Here's how the part is built. I have some questions about the finished solid (model axes, mm). A direction names the side the tool comes from. Coordinates: 2 decimals unless noted, no trailing zeros. Order: outer loops, then holes, each group sorted by start corner. A loop starts at its lowest first (then second) coordinate and runs counter-clockwise, first axis right, second up. Notation, with made-up numbers: (-1, 43.5) - (55, 43.5) arc R17 cw to (55, 52.5) - close; hole circle Ø3 at (84, 29.25). An arc over 180 degrees is marked (long way). Answer in a Markdown table with one row per item. Add a question column.
Item 1: Thinking about a two-plate mould opening in X: for faces 4 (the flat face through (42, 1, -32.5)), 5 (the flat face through (19, 1, -30)), 6 (the cylindrical face through (47.657, 1.47, -40.52)), which applies, +X half, -X half, draft (parallel to the pull), parting line (faces both ways), or undercut?
Item 2: I want a section at B-B (x = -24). Please give me the cut outline in (y, z), plus the area to 3 significant figures.
Item 3: Will these pins go through, and if not, where does the flat tip stop? pin 1 Ø7.5 at (x, z) = (50, -40) entering from +Y; pin 2 Ø0.9 at (x, y) = (35, 1) entering from +Z; pin 3 Ø0.9 at (y, z) = (1, -34) entering from +X; pin 4 Ø1.5 at (x, y) = (20, 2) entering from -Z.
Item 4: I want a section at C-C (y = 1.15). Please give me the cut outline in (x, z).
Item 5: If I drill on line 1 along X through (y, z) = (2.45, -46.5); line 2 along X through (y, z) = (1.15, -53); line 3 along X through (y, z) = (2.7, -38), over which ranges is the centre line in solid material (lowest first)? Write a range as from..to.
Item 6: On a 3-axis mill with a long thin cutter (end or side, diameter ignored), from which of +Z, -Z, +X, -X, +Y, -Y can I reach the whole of each face in a straight line? I mean faces 1 (the flat face through (0, 1, -45.2)), 2 (the cylindrical face through (1.13, 1.43, -72.99)), 3 (the flat face through (-43, 1, -32.5)). Say none if no direction works.
Item 7: I want a section at D-D (z = -40.5). Please give me the cut outline in (x, y), plus the area to 3 significant figures.
Item 8: I want a section at A-A (z = -48). Please give me the cut outline in (x, y).
```python
from build123d import *

# Parameters (mm, degrees)
BOSS_EXTRUDE1_DEPTH  = 2.9
SOLENOID_PLACEMENT_W = 38
SOLENOID_PLACEMENT_H = 64
CUT_EXTRUDE1_DEPTH   = 104.278313309
CUT_EXTRUDE4_DEPTH   = 104.278313309
SKETCH5_R            = 12
CUT_EXTRUDE5_DEPTH   = 104.278313309
SKETCH6_R            = 2.4
CUT_EXTRUDE6_DEPTH   = 104.278313309
CUT_EXTRUDE3_DEPTH   = 104.278313309


with BuildPart() as part:
    # Sketch1 → Boss-Extrude1 (new body)
    with BuildSketch(Plane(origin=(0, 0, 0), x_dir=(1, 0, 0), z_dir=(0, 1, 0))):
        with BuildLine():
            ThreePointArc((36.856602833, -63.012624351), (0, 73), (-36.856602833, -63.012624351))
            ThreePointArc((-36.856602833, -63.012624351), (-33.368752207, -63.602994345), (-30.363140064, -61.737536127))
            ThreePointArc((-30.363140064, -61.737536127), (0, -46.75), (30.363140064, -61.737536127))
            ThreePointArc((30.363140064, -61.737536127), (33.368752207, -63.602994345), (36.856602833, -63.012624351))
        make_face()
    extrude(amount=BOSS_EXTRUDE1_DEPTH)

    # solenoid placement → Cut-Extrude1 (cut, through all)
    with BuildSketch(Plane(origin=(0, 2.9, 0), x_dir=(1, 0, 0), z_dir=(0, 1, 0))):
        with Locations((0, -4)):
            Rectangle(SOLENOID_PLACEMENT_W, SOLENOID_PLACEMENT_H)
    extrude(amount=-CUT_EXTRUDE1_DEPTH, mode=Mode.SUBTRACT)

    # Sketch4 → Cut-Extrude4 (cut, through all)
    with BuildSketch(Plane(origin=(0, 2.9, 0), x_dir=(1, 0, 0), z_dir=(0, 1, 0))):
        with BuildLine():
            Line((-13, 28), (13, 28))
            Line((13, 28), (13, 43.2))
            ThreePointArc((13, 43.2), (12.414213562, 44.614213562), (11, 45.2))
            Line((11, 45.2), (-11, 45.2))
            ThreePointArc((-11, 45.2), (-12.414213562, 44.614213562), (-13, 43.2))
            Line((-13, 43.2), (-13, 28))
        make_face()
    extrude(amount=-CUT_EXTRUDE4_DEPTH, mode=Mode.SUBTRACT)

    # Sketch5 → Cut-Extrude5 (cut, through all)
    with BuildSketch(Plane(origin=(0, 2.9, 0), x_dir=(1, 0, 0), z_dir=(0, 1, 0))):
        with Locations(Location((-27, 48, 0), (0, 0, 270))):
            Circle(SKETCH5_R)
        with Locations(Location((27, 48, 0), (0, 0, 270))):
            Circle(SKETCH5_R)
    extrude(amount=-CUT_EXTRUDE5_DEPTH, mode=Mode.SUBTRACT)

    # Sketch6 → Cut-Extrude6 (cut, through all)
    with BuildSketch(Plane(origin=(0, 2.9, 0), x_dir=(1, 0, 0), z_dir=(0, 1, 0))):
        with Locations(Location((40, -40, 0), (0, 0, 270))):
            Circle(SKETCH6_R)
        with Locations(Location((-40, -40, 0), (0, 0, 270))):
            Circle(SKETCH6_R)
        with Locations(Location((-50, 40, 0), (0, 0, 270))):
            Circle(SKETCH6_R)
        with Locations(Location((50, 40, 0), (0, 0, 270))):
            Circle(SKETCH6_R)
    extrude(amount=-CUT_EXTRUDE6_DEPTH, mode=Mode.SUBTRACT)

    # Sketch3 → Cut-Extrude3 (cut, through all)
    with BuildSketch(Plane(origin=(0, 2.9, 0), x_dir=(1, 0, 0), z_dir=(0, 1, 0))):
        Polygon((-19, 28), (19, 28), (19, 32.5), (73, 32.5), (73, -32.5), (-73, -32.5), (-73, 32.5), (-19, 32.5), align=None)
    extrude(amount=-CUT_EXTRUDE3_DEPTH, mode=Mode.SUBTRACT)


with BuildPart() as cut_extrude3_piece_1:
    # of the separate pieces the step leaves, piece 1, a body of its own (cut_extrude3_pieces)
    add(part.part.solids().sort_by_distance((65.366275709, 0, -32.5))[0])


with BuildPart() as cut_extrude3_piece_2:
    # of the separate pieces the step leaves, piece 2, a body of its own (cut_extrude3_pieces)
    add(part.part.solids().sort_by_distance((-36.856602833, 0, 63.012624351))[0])


solid = cut_extrude3_piece_1.part
```
Values follow:
| question | item | result |
|---|---|---|
| 1 | face 4 | draft |
| 1 | face 5 | +X half |
| 1 | face 6 | undercut |
| 2 | outline | (0, -68.94) - (2.9, -68.94) - (2.9, -59.62) - (0, -59.62) - close; (0, -36.38) - (2.9, -36.38) - (2.9, -32.5) - (0, -32.5) - close |
| 2 | area | 38.3 mm^2 |
| 3 | pin 1 | stops at y = 2.9 |
| 3 | pin 2 | stops at z = -32.5 |
| 3 | pin 3 | stops at x = 64.83 |
| 3 | pin 4 | stops at z = -70.42 |
| 4 | outline | (-65.37, -32.5) arc R73 ccw to (65.37, -32.5) - (19, -32.5) - (19, -28) - (13, -28) - (13, -43.2) arc R2 cw to (11, -45.2) - (-11, -45.2) arc R2 cw to (-13, -43.2) - (-13, -28) - (-19, -28) - (-19, -32.5) - close; hole circle Ø4.8 at (-50, -40); hole circle Ø24 at (-27, -48); hole circle Ø24 at (27, -48); hole circle Ø4.8 at (50, -40) |
| 5 | line 1 | x = -56.27..-38.91, -15.09..15.09, 38.91..56.27 |
| 5 | line 2 | x = -50.2..-37.91, -16.09..16.09, 37.91..50.2 |
| 5 | line 3 | x = -62.33..-51.33, -48.67..-33.63, -20.37..-13, 13..20.37, 33.63..48.67, 51.33..62.33 |
| 6 | face 1 | +Z, +Y, -Y |
| 6 | face 2 | -Z, +Y, -Y |
| 6 | face 3 | +Z, -X, +Y, -Y |
| 7 | outline | (-60.74, 0) - (-52.35, 0) - (-52.35, 2.9) - (-60.74, 2.9) - close; (-47.65, 0) - (-36.37, 0) - (-36.37, 2.9) - (-47.65, 2.9) - close; (-17.63, 0) - (-13, 0) - (-13, 2.9) - (-17.63, 2.9) - close; (13, 0) - (17.63, 0) - (17.63, 2.9) - (13, 2.9) - close; (36.37, 0) - (47.65, 0) - (47.65, 2.9) - (36.37, 2.9) - close; (52.35, 0) - (60.74, 0) - (60.74, 2.9) - (52.35, 2.9) - close |
| 7 | area | 141 mm^2 |
| 8 | outline | (-55, 0) - (-39, 0) - (-39, 2.9) - (-55, 2.9) - close; (-15, 0) - (15, 0) - (15, 2.9) - (-15, 2.9) - close; (39, 0) - (55, 0) - (55, 2.9) - (39, 2.9) - close |
